from build123d import *
from build123d.topology import SkipClean

# Parameters (mm, degrees)
LEFT_ARM_DEPTH                = 12.5
SKETCH2_R                     = 20
LEFT_BOSS_DEPTH               = 37.5
LEFT_HEX_DEPTH                = 237.801604724
LEFT_HEX_DEPTH_BACK           = 237.801604724
SKETCH3_R                     = 65
CENTRE_BOSS_DEPTH             = 35
SKETCH5_W                     = 25
SKETCH5_H                     = 40
RIGHT_ARM_DEPTH               = 180
SKETCH7_R                     = 30
RIGHT_BOSS_DEPTH              = 37.5
SKETCH8_R                     = 17.5
RIGHT_BOSS_HOLE_DEPTH         = 369.660954503
SKETCH9_R                     = 40
CENTRE_HOLE_DEPTH             = 369.160494044
SKETCH10_R                    = 27.5
CENTRE_BLOB_DEPTH             = 35
CENTRE_BEAM_REACH             = 224.371
SKETCH11_W                    = 10
SKETCH11_H                    = 30
CENTRE_BEAM_DIRECTION_2_REACH = 224.371
SKETCH12_R                    = 20
CUT_EXTRUDE4_DEPTH            = 5
M6X1_0_TAPPED_HOLE1_D         = 5
CIRPATTERN1_COUNT             = 6
CUT_OUT_DEPTH                 = 10
FILLET1_R                     = 10
FILLET1_OF_MIRROR2_R          = 10
KEYWAY_DEPTH                  = 363.894129706


with BuildPart() as part:
    # Sketch1 → LEFT_ARM (new, symmetric)
    with BuildSketch(Plane.XY):
        with BuildLine():
            Line((-6, 19.078784028), (130.5, 62.006048092))
            ThreePointArc((130.5, 62.006048092), (215, 0), (130.5, -62.006048092))
            Line((130.5, -62.006048092), (-6, -19.078784028))
            ThreePointArc((-6, -19.078784028), (-20, 0), (-6, 19.078784028))
        make_face()
    extrude(amount=LEFT_ARM_DEPTH, both=True)

    # Sketch2 → LEFT_Boss (add, symmetric)
    with SkipClean():  # the faces are left unmerged after this step: merging them gives an invalid solid
        with BuildSketch(Plane.XY):
            Circle(SKETCH2_R)
        extrude(amount=LEFT_BOSS_DEPTH, both=True)

    # Sketch4 → LEFT_Hex (cut, two sides: drawn at the far end of the back side and taken through both)
    with SkipClean():  # the faces are left unmerged after this step: merging them gives an invalid solid
        with BuildSketch(Plane.XY.offset(37.5).offset(-LEFT_HEX_DEPTH_BACK)):
            Polygon((14.43375673, 0), (7.216878365, 12.5), (-7.216878365, 12.5), (-14.43375673, 0), (-7.216878365, -12.5), (7.216878365, -12.5), align=None)
        extrude(amount=LEFT_HEX_DEPTH + LEFT_HEX_DEPTH_BACK, mode=Mode.SUBTRACT)

    # Sketch3 → CENTRE_Boss (add, symmetric)
    with SkipClean():  # the faces are left unmerged after this step: merging them gives an invalid solid
        with BuildSketch(Plane.XY):
            with Locations((150, 0)):
                Circle(SKETCH3_R)
        extrude(amount=CENTRE_BOSS_DEPTH, both=True)

    # Sketch5 → RIGHT_ARM (add)
    with SkipClean():  # the faces are left unmerged after this step: merging them gives an invalid solid
        with BuildSketch(Plane(origin=(132.453333234, 48.209070726, 0), x_dir=(0, 0, -1), z_dir=(0.9396926207859081, 0.34202014332566943, 0))):
            with Locations((0, -51.303021499)):
                Rectangle(SKETCH5_W, SKETCH5_H)
        extrude(amount=RIGHT_ARM_DEPTH)

    # Sketch7 → RIGHT_Boss (add, symmetric)
    with SkipClean():  # the faces are left unmerged after this step: merging them gives an invalid solid
        with BuildSketch(Plane.XY):
            with Locations((319.144671741, 61.563625799)):
                Circle(SKETCH7_R)
        extrude(amount=RIGHT_BOSS_DEPTH, both=True)
    add(part.part.scale(1), mode=Mode.REPLACE)  # the faces are merged on a copy

    # Sketch8 → RIGHT_Boss_Hole (cut, through all)
    with BuildSketch(Plane.XY.offset(37.5)):
        with Locations((319.144671741, 61.563625799)):
            Circle(SKETCH8_R)
    extrude(amount=-RIGHT_BOSS_HOLE_DEPTH, mode=Mode.SUBTRACT)

    # Sketch9 → CENTRE_Hole (cut, through all)
    with BuildSketch(Plane.XY.offset(35)):
        with Locations((150, 0)):
            Circle(SKETCH9_R)
    extrude(amount=-CENTRE_HOLE_DEPTH, mode=Mode.SUBTRACT)

    # Sketch10 → CENTRE_Blob (add, symmetric)
    with SkipClean():  # the faces are left unmerged after this step: merging them gives an invalid solid
        with BuildSketch(Plane.XY):
            with Locations((173.49231552, 8.550503583)):
                Circle(SKETCH10_R)
        extrude(amount=CENTRE_BLOB_DEPTH, both=True)

    # Sketch11 → CENTRE_Beam (add, up to next)
    with BuildSketch(Plane(origin=(150, 0, 0), x_dir=(0, 0, -1), z_dir=(1, 0, 0)), mode=Mode.PRIVATE) as centre_beam_sk1:
        Rectangle(SKETCH11_W, SKETCH11_H)
    centre_beam_tool1 = extrude(centre_beam_sk1.sketch, amount=CENTRE_BEAM_REACH, mode=Mode.PRIVATE) - part.part
    add(centre_beam_tool1.solids().sort_by_distance((150, 0, 0))[0])

    # Sketch11 → CENTRE_Beam direction 2 (add, up to next)
    with BuildSketch(Plane(origin=(150, 0, 0), x_dir=(0, 0, -1), z_dir=(1, 0, 0)), mode=Mode.PRIVATE) as centre_beam_direction_2_sk1:
        Rectangle(SKETCH11_W, SKETCH11_H)
    centre_beam_direction_2_tool1 = extrude(centre_beam_direction_2_sk1.sketch, amount=-CENTRE_BEAM_DIRECTION_2_REACH, mode=Mode.PRIVATE) - part.part
    add(centre_beam_direction_2_tool1.solids().sort_by_distance((150, 0, 0))[0])

    # Sketch12 → Cut-Extrude4 (cut)
    with BuildSketch(Plane.XY.offset(35)):
        with Locations((173.49231552, 8.550503583)):
            Circle(SKETCH12_R)
    cut_extrude4 = extrude(amount=-CUT_EXTRUDE4_DEPTH, mode=Mode.SUBTRACT)

    # M6x1.0 Tapped Hole1 (through all)
    with Locations(Plane.XY.offset(30)):
        with Locations((159.396926208, 3.420201433)):
            m6x1_0_tapped_hole1 = Hole(M6X1_0_TAPPED_HOLE1_D / 2)

    # CirPattern1: M6x1.0 Tapped Hole1 ×6 about axis
    cirpattern1_axis = Axis((173.49231552, 8.550503583, 0), (0, 0, 1))
    for i in range(1, CIRPATTERN1_COUNT):
        add(m6x1_0_tapped_hole1.rotate(cirpattern1_axis, i * 360 / CIRPATTERN1_COUNT), mode=Mode.SUBTRACT)

    # Mirror1: Cut-Extrude4 across plane
    add(cut_extrude4.mirror(Plane.XY), mode=Mode.SUBTRACT)

    # Sketch15 → Cut_OUT (cut)
    with BuildSketch(Plane.XY.offset(12.5)):
        with BuildLine():
            Line((84.858453972, 37.169597537), (23.981475126, 18.024673388))
            ThreePointArc((23.981475126, 18.024673388), (30, 0), (23.981475126, -18.024673388))
            Line((23.981475126, -18.024673388), (84.858453972, -37.169597537))
            ThreePointArc((84.858453972, -37.169597537), (75, 0), (84.858453972, 37.169597537))
        make_face()
    cut_out = extrude(amount=-CUT_OUT_DEPTH, mode=Mode.SUBTRACT)

    # Fillet1
    fillet1_edges = [part.edges().sort_by_distance(p)[0] for p in [
        (23.981475126, -18.024673388, 7.5),
        (23.981475126, 18.024673388, 7.5),
        (84.858453972, 37.169597537, 7.5),
        (84.858453972, -37.169597537, 7.5),
    ]]
    fillet(fillet1_edges, radius=FILLET1_R)

    # Mirror2: Cut_OUT across plane
    with SkipClean():  # the faces are left unmerged after this step: merging them gives an invalid solid
        add(cut_out.mirror(Plane.XY), mode=Mode.SUBTRACT)

    # Fillet1 of Mirror2
    fillet1_of_mirror2_edges = [part.edges().sort_by_distance(p)[0] for p in [
        (23.981475126, -18.024673388, -7.5),
        (23.981475126, 18.024673388, -7.5),
        (84.858453972, 37.169597537, -7.5),
        (84.858453972, -37.169597537, -7.5),
    ]]
    fillet(fillet1_of_mirror2_edges, radius=FILLET1_OF_MIRROR2_R)

    # Sketch16 → KEYWAY (cut, symmetric)
    with SkipClean():  # the faces are left unmerged after this step: merging them gives an invalid solid
        with BuildSketch(Plane.XY):
            Polygon((320.854772458, 56.865162695), (317.434571025, 66.262088903), (297.888964512, 59.148069921), (301.309165946, 49.751143714), align=None)
        keyway = extrude(amount=KEYWAY_DEPTH, both=True, mode=Mode.SUBTRACT)

    # Mirror3: KEYWAY across plane
    with SkipClean():  # the faces are left unmerged after this step: merging them gives an invalid solid
        add(keyway.mirror(Plane(origin=(301.598004975, 109.772696525, 0), x_dir=(0, 0, 1), z_dir=(0.9396926207859081, 0.34202014332566943, 0))), mode=Mode.SUBTRACT)


solid = part.part
Verification items for the finished model (mm, model axes). A direction names the side the tool comes from. Coordinates: 2 decimals unless noted, no trailing zeros. Order: outer loops, then holes, each group sorted by start corner. A loop starts at its lowest first (then second) coordinate and runs counter-clockwise, first axis right, second up. Notation, with made-up numbers: M -17,-28 L 15,-28 A25 cw 15,-13 Z; hole C 72,14 d2. An arc over 180 degrees is marked long. Return JSON: item names as keys, results as strings.
1) Release check for a two-part mould opening along Y. For faces 1 (the cylindrical face through (347.76, 70.57, 0.52)), 2 (the flat face through (50.14, 26.25, 7.57)), 3 (the flat face through (253, 37, 12.5)) record: +Y half, -Y half, draft (parallel to the pull), parting line (faces both ways), or undercut.
Answer list:
{"face 1": "parting line", "face 2": "undercut", "face 3": "draft"}
2) Thickness scan on L1, parallel to X at y = 57, z = 32.5; L2, parallel to X at y = -16.5, z = -2; L3, parallel to X at y = -4, z = -23. Record the ranges inside material, lowest first. Write a range as [from, to].
Answer list:
{"L1": "[118.76, 181.24], [289.49, 298.67], [336.04, 348.8]", "L2": "[-11.3, 113.56], [162.15, 184.84], [186.44, 212.87]", "L3": "[-19.6, -12.12], [12.12, 19.6], [85.12, 110.2], [149.02, 169.74], [172.03, 214.88]"}
3) Access from +Z, -Z, +X, -X, +Y, -Y to the whole of each face (thin tool, end or side, straight path). Record for faces 4 (the cylindrical face through (74.704, -28.441, -7.43)), 5 (the flat face through (130, 0, 5)), 6 (the flat face through (130, 15, 0)), 7 (the flat face through (149, 1, -35)).
Answer list:
{"face 4": "-Z", "face 5": "+Z", "face 6": "+Z, -Z", "face 7": "-Z, +Y, -Y"}
4) Cross-section at B-B, the plane x = 59. Record the boundary of the cut face in (y, z), and give its area (3 significant figures).
Answer list:
{"outline": "M -39.52,-12.5 L -29.04,-12.5 L -29.04,-2.5 L 29.04,-2.5 L 29.04,-12.5 L 39.52,-12.5 L 39.52,12.5 L 29.04,12.5 L 29.04,2.5 L -29.04,2.5 L -29.04,12.5 L -39.52,12.5 Z", "area": "815 mm2"}
5) Gauge pin test, flat ends, axial feed: pin 1 (8 mm diameter, centred on x = 94.5, y = 50.5, fed in from -Z); pin 2 (7 mm diameter, centred on x = 0, z = -15.5, fed in from +Y); pin 3 (10 mm diameter, centred on x = 234.5, y = 11.5, fed in from +Z). Record the tip position at first contact, or that the pin passes through.
Answer list:
{"pin 1": "z = -12.5", "pin 2": "y = 21.53", "pin 3": "z = 12.5"}
6) Cross-section at C-C, the plane x = 275. Record the boundary of the cut face in (y, z).
Answer list:
{"outline": "M 24.21,-12.5 L 66.78,-12.5 L 66.78,12.5 L 24.21,12.5 Z"}
7) Cross-section at A-A, the plane x = 0. Record the boundary of the cut face in (y, z).
Answer list:
{"outline": "M -20.97,-12.5 L -20,-12.5 L -20,-37.5 L -12.5,-37.5 L -12.5,37.5 L -20,37.5 L -20,12.5 L -20.97,12.5 Z; M 12.5,-37.5 L 20,-37.5 L 20,-12.5 L 20.97,-12.5 L 20.97,12.5 L 20,12.5 L 20,37.5 L 12.5,37.5 Z"}
